Geometry: final body of the model. Coordinates: model frame, mm. A direction names the side the tool comes from. Coordinates: 2 decimals unless noted, no trailing zeros. Loops run counter-clockwise (first coordinate to the right, second up) from the corner with the lowest first, then second, coordinate; pieces in that order, holes last. Notation, with made-up numbers: M 75.25,37.25 L 85.25,37.25 A26 cw 85.25,75.25 Z; hole C -4,75 d2. An arc over 180 degrees is marked long. Write each question's results on one line, items separated by ' | '. Start each with the question number.
from build123d import *

# Parameters (mm, degrees)
F0_W     = 89.4021987915
F0_H     = 75.7953710854
F2_DEPTH = 117.856964469
F3_W     = 76.7021987915
F3_H     = 63.0953710854
F4_DEPTH = 168.5473639518
F6_DEPTH = 108.4326226264


with BuildPart() as f2:
    # F0 (on Right) → F2 (new body)
    with BuildSketch(Plane.YZ):
        with Locations((44.7010993958, 4.8550125211)):
            Rectangle(F0_W, F0_H)
    extrude(amount=F2_DEPTH)

    # F3 (on face) → F4 (cut)
    with BuildSketch(Plane.YZ.offset(117.856964469)):
        with Locations((44.7010993958, 4.8550125211)):
            Rectangle(F3_W, F3_H)
    extrude(amount=-F4_DEPTH, mode=Mode.SUBTRACT)

    # F5 (on face) → F6 (cut)
    with BuildSketch(Plane.XZ):
        Polygon((70.9031159894, -18.7701933731), (80.4803622858, 5.5882447229), (60.2736428727, 22.2239185493), (38.2079571779, 8.1468923038), (44.7773328466, -17.1888622029), align=None)
    extrude(amount=-F6_DEPTH, mode=Mode.SUBTRACT)


solid = f2.part
Item 1: Set-up query: faces 5 (the flat face through (58, 44, 42.753)), 6 (the flat face through (73, 83.052, 18)), 7 (the flat face through (41.447, 86.183, -4.344)). Return all of +Z, -Z, +X, -X, +Y, -Y with unobstructed straight access to the full face (end or side cutting, diameter ignored); none if empty.
Item 2: Section D-D, the plane z = -9. Return loops of the section in (x, y).
Item 3: Section A-A, the plane y = 53. Return loops of the section in (x, z).
Item 4: Contact query for a flat-ended pin moving along its axis: P1, Ø19, axis at x = 75, z = -6, coming from the -Y side. Output: stop coordinate, or through.
Item 5: Section C-C, the plane x = 21. Return loops of the section in (y, z).
Item 6: Section B-B, the plane z = 24. Return loops of the section in (x, y), plus the area to 3 significant figures.
Item 7: Pull-direction query (Y, two-part tool) for faces 1 (the flat face through (60, 44, -26.693)), 2 (the flat face through (45, 89.402, 13)), 3 (the flat face through (45, 0, 13)), 4 (the flat face through (75.625, 86.183, -6.761)); classes: released by +Y, released by -Y, zero draft, split by the parting line, or undercut.
Item 8: Ray query, L1, parallel to Y at x = 33.5, z = 25.5; L2, parallel to Z at x = 96, y = 77; L3, parallel to X at y = 83.5, z = 5. Return the intervals inside material, ascending. Write a range as [from, to].
Solutions:
1) face 5: +Z, +X, -X, +Y, -Y | face 6: +X, -X | face 7: +Y, -Y
2) outline: M 0,0 L 42.65,0 L 42.65,6.35 L 0,6.35 Z; M 0,83.05 L 42.65,83.05 L 42.65,89.4 L 0,89.4 Z; M 74.74,0 L 117.86,0 L 117.86,6.35 L 74.74,6.35 Z; M 74.74,83.05 L 117.86,83.05 L 117.86,89.4 L 74.74,89.4 Z
3) outline: M 0,-33.04 L 117.86,-33.04 L 117.86,-26.69 L 0,-26.69 Z; M 0,36.4 L 117.86,36.4 L 117.86,42.75 L 0,42.75 Z
4) P1: stops at y = 0
5) outline: M 0,-33.04 L 89.4,-33.04 L 89.4,42.75 L 0,42.75 Z; hole M 6.35,-26.69 L 83.05,-26.69 L 83.05,36.4 L 6.35,36.4 Z
6) outline: M 0,0 L 117.86,0 L 117.86,6.35 L 0,6.35 Z; M 0,83.05 L 117.86,83.05 L 117.86,89.4 L 0,89.4 Z | area: 1,500 mm²
7) face 1: undercut | face 2: released by +Y | face 3: released by -Y | face 4: zero draft
8) L1: y = [0, 6.35], [83.05, 89.4] | L2: z = [-33.04, -26.69], [36.4, 42.75] | L3: x = [0, 39.02], [80.25, 117.86]
